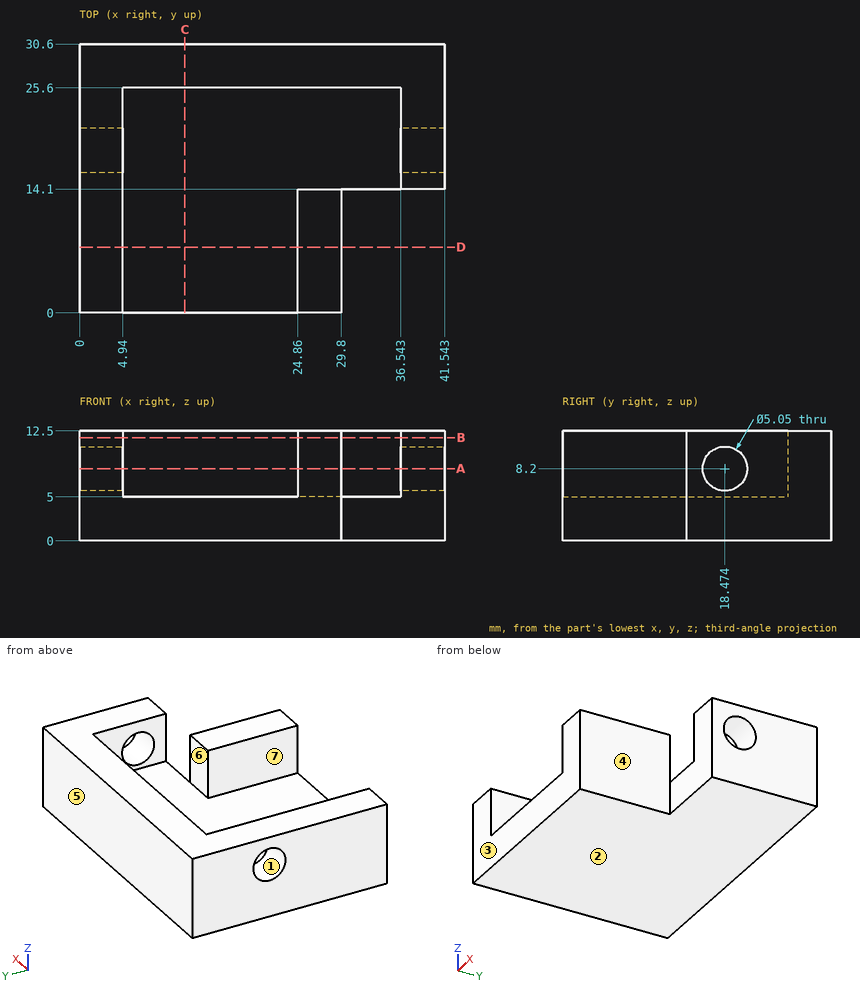
Study the drawing (mm; zero at the part's minimum x, y, z) and answer. A direction names the side the tool comes from. Coordinates: 2 decimals unless noted, no trailing zeros. Write each loop counter-clockwise with the first axis right and the second up, starting at its lowest first coordinate (ties: lowest second). Pieces come first, ordered by that corner, then holes. Notation, with made-up numbers: (19, -2.75) -> (70, -2.75) arc R21 cw to (70, 36.25) -> close; hole circle Ø5 at (81.5, -15). An arc over 180 degrees is marked (long way). Write each question's results on one line, items separated by ' | '. Start each with the question number.
1) Straight lines are drawn through the part: probe 1 along X at (y, z) = (12, 11.75); probe 2 along Y at (x, z) = (2.3, 8.2); probe 3 along X at (y, z) = (16, 6.75). For each, find the intervals that lie inside material, in ascending order.
2) A cutting plane is placed at A-A (z = 8.2). Determine the outline of the cut face in (x, y), then the cut area to 3 significant figures.
3) A tool of negligible diameter and unlimited length cuts with its end or side. For the marked faces 4, 5, 6 and 7, from which of +Z, -Z, +X, -X, +Y, -Y can it reach the whole face along a straight path? Write none if from no direction.
4) For a pull along Z with two mould halves and no side action, classify the marked faces 1, 2 and 3 as +Z half, -Z half, draft (parallel to the pull), parting line (faces both ways), or undercut.
5) A cutting plane is placed at C-C (x = 12). Determine the outline of the cut face in (y, z).
6) A cutting plane is placed at D-D (y = 7.5). Determine the outline of the cut face in (x, z).
7) Flat-ended cylindrical pins translate along their axes: pin 1 Ø10 at (x, y) = (35, 6.5) entering from +Z; pin 2 Ø1 at (y, z) = (6.5, 5.5) entering from +X. Find the tip coordinate at first contact, or state that the pin passes through.
8) A cutting plane is placed at B-B (z = 11.75). Determine the outline of the cut face in (x, y).
Values follow:
1) probe 1: 0 to 4.94, 24.86 to 29.8 | probe 2: 0 to 15.95, 21 to 30.6 | probe 3: 0 to 4.94, 36.54 to 41.54
2) outline: (0, 0) -> (4.94, 0) -> (4.94, 15.95) -> (0, 15.95) -> close; (0, 21) -> (4.94, 21) -> (4.94, 25.6) -> (36.54, 25.6) -> (36.54, 21) -> (41.54, 21) -> (41.54, 30.6) -> (0, 30.6) -> close; (24.86, 0) -> (29.8, 0) -> (29.8, 14.1) -> (24.86, 14.1) -> close; (36.54, 14.1) -> (41.54, 14.1) -> (41.54, 15.95) -> (36.54, 15.95) -> close | area: 411 mm²
3) face 4: +Z, -Z, +X, -Y | face 5: +Z, -Z, +X, -X, +Y | face 6: +Z | face 7: +Z, -Y
4) face 1: undercut | face 2: -Z half | face 3: draft
5) outline: (0, 0) -> (30.6, 0) -> (30.6, 12.5) -> (25.6, 12.5) -> (25.6, 5) -> (0, 5) -> close
6) outline: (0, 0) -> (29.8, 0) -> (29.8, 12.5) -> (24.86, 12.5) -> (24.86, 5) -> (4.94, 5) -> (4.94, 12.5) -> (0, 12.5) -> close
7) pin 1: through | pin 2: x = 29.8
8) outline: (0, 0) -> (4.94, 0) -> (4.94, 25.6) -> (36.54, 25.6) -> (36.54, 14.1) -> (41.54, 14.1) -> (41.54, 30.6) -> (0, 30.6) -> close; (24.86, 0) -> (29.8, 0) -> (29.8, 14.1) -> (24.86, 14.1) -> close
